Read the model definition and answer for the solid it produces. Units are mm, in the model's axes. Coordinates: 2 decimals unless noted, no trailing zeros. Write each loop counter-clockwise with the first axis right and the second up, starting at its lowest first coordinate (ties: lowest second). Pieces come first, ordered by that corner, then holes. Notation, with made-up numbers: (-1, -17) -> (10, -17) arc R18 cw to (10, 11) -> close; hole circle Ø6 at (50, 52.5). An arc over 180 degrees is marked (long way). Answer in a Markdown table with one row per item. Add a question column.
Item 1: Section A-A on z = 4.25 is taken. Count the separate pieces of the cut face and the enclosed holes in it, then the cut area to 3 significant figures.
Item 2: Section B-B on x = -21 is taken. Write down the section's boundary in (y, z), then the cut area to 3 significant figures.
Item 3: For a pull along X with two mould halves and no side action, classify faces 1 (the face through (-8.67, -39.05, 2.46)), 2 (the face through (-1, -8, 5)), 3 (the face through (0, -13, 3)) as +X half, -X half, draft (parallel to the pull), parting line (faces both ways), or undercut.
Item 4: Given pin 1 Ø1.5 at (y, z) = (-24, 3) entering from -X; pin 2 Ø1.5 at (x, z) = (-22.5, 2.5) entering from +Y; pin 3 Ø1 at (x, z) = (28.5, 1.5) entering from -Y, each flat-ended and moving along its own axis, determine where each tip first touches the part or whether it passes through.
Item 5: Section C-C on y = -18 is taken. Write down the section's boundary in (x, z).
Item 6: Straight lines are drawn through the part: line 1 (Y direction, x = 0, z = 1.7); line 2 (X direction, y = -19, z = 0.95); line 3 (X direction, y = -19.5, z = 4.6). For each, find the intervals that lie inside material, in ascending order. Write a range as from..to.
Item 7: Section D-D on y = -36 is taken. Write down the section's boundary in (x, z), then the cut area to 3 significant figures.
```python
from build123d import *

# Parameters (mm, degrees)
SKETCH1_R           = 40
SKETCH1_R_2         = 0.75
BOSS_EXTRUDE1_DEPTH = 5
SKETCH4_W           = 10
SKETCH4_H           = 15
SKETCH4_W_2         = 15
SKETCH4_H_2         = 10
CUT_EXTRUDE3_DEPTH  = 6
SKETCH5_R           = 1.7
CUT_EXTRUDE4_DEPTH  = 6
SKETCH6_R           = 0.85
CUT_EXTRUDE5_DEPTH  = 6


with BuildPart() as part:
    # Sketch1 → Boss-Extrude1 (new body)
    with BuildSketch(Plane.XY):
        Circle(SKETCH1_R)
        Circle(SKETCH1_R_2, mode=Mode.SUBTRACT)
    extrude(amount=BOSS_EXTRUDE1_DEPTH)

    # Sketch4 → Cut-Extrude3 (cut, through all)
    with BuildSketch(Plane.XY.offset(5)):
        with Locations((0, 20.5)):
            Rectangle(SKETCH4_W, SKETCH4_H)
        with Locations((20.5, 0)):
            Rectangle(SKETCH4_W_2, SKETCH4_H_2)
        with Locations((0, -20.5)):
            Rectangle(SKETCH4_W, SKETCH4_H)
        with Locations((-20.5, 0)):
            Rectangle(SKETCH4_W_2, SKETCH4_H_2)
    extrude(amount=-CUT_EXTRUDE3_DEPTH, mode=Mode.SUBTRACT)

    # Sketch5 → Cut-Extrude4 (cut, through all)
    with BuildSketch(Plane.XY.offset(5)):
        with Locations((0, 36)):
            Circle(SKETCH5_R)
        with Locations((31.176914536, 18)):
            Circle(SKETCH5_R)
        with Locations((31.176914536, -18)):
            Circle(SKETCH5_R)
        with Locations((0, -36)):
            Circle(SKETCH5_R)
        with Locations((-31.176914536, -18)):
            Circle(SKETCH5_R)
        with Locations((-31.176914536, 18)):
            Circle(SKETCH5_R)
    extrude(amount=-CUT_EXTRUDE4_DEPTH, mode=Mode.SUBTRACT)

    # Sketch6 → Cut-Extrude5 (cut, through all)
    with BuildSketch(Plane.XY.offset(5)):
        Circle(SKETCH6_R)
    extrude(amount=-CUT_EXTRUDE5_DEPTH, mode=Mode.SUBTRACT)


solid = part.part
```
Results below:
| question | item | result |
|---|---|---|
| 1 | separate pieces | 1 |
| 1 | enclosed holes | 11 |
| 1 | area | 4,370 mm2 |
| 2 | outline | (-34.04, 0) -> (-5, 0) -> (-5, 5) -> (-34.04, 5) -> close; (5, 0) -> (34.04, 0) -> (34.04, 5) -> (5, 5) -> close |
| 2 | area | 290 mm2 |
| 3 | face 1 | parting line |
| 3 | face 2 | draft |
| 3 | face 3 | undercut |
| 4 | pin 1 | stops at x = -32.55 |
| 4 | pin 2 | stops at y = 33.57 |
| 4 | pin 3 | stops at y = -28.57 |
| 5 | outline | (-35.72, 0) -> (-32.88, 0) -> (-32.88, 5) -> (-35.72, 5) -> close; (-29.48, 0) -> (-5, 0) -> (-5, 5) -> (-29.48, 5) -> close; (5, 0) -> (29.48, 0) -> (29.48, 5) -> (5, 5) -> close; (32.88, 0) -> (35.72, 0) -> (35.72, 5) -> (32.88, 5) -> close |
| 6 | line 1 | y = -40..-37.7, -34.3..-28, -13..-0.85, 0.85..13, 28..34.3, 37.7..40 |
| 6 | line 2 | x = -35.2..-32.55, -29.8..-5, 5..29.8, 32.55..35.2 |
| 6 | line 3 | x = -34.92..-31.98, -30.38..-5, 5..30.38, 31.98..34.92 |
| 7 | outline | (-17.44, 0) -> (-1.7, 0) -> (-1.7, 5) -> (-17.44, 5) -> close; (1.7, 0) -> (17.44, 0) -> (17.44, 5) -> (1.7, 5) -> close |
| 7 | area | 157 mm2 |
